```python
from build123d import *

# Parameters (mm, degrees)
SKETCH1_R               = 12.9794
BOSS_EXTRUDE1_DEPTH     = 25.4
CUT_EXTRUDE1_DEPTH      = 76.208452105
CUT_EXTRUDE1_DEPTH_BACK = 76.208452105
SKETCH3_R               = 3.81
SKETCH6_R               = 8.255
CUT_EXTRUDE2_DEPTH      = 2.032
SKETCH7_R               = 3.81
SKETCH7_R_2             = 1.905
CUT_EXTRUDE3_DEPTH      = 26.67
SKETCH7_3_R             = 1.905
CUT_EXTRUDE4_DEPTH      = 46.693656372


with BuildPart() as part:
    # Sketch1 → Boss-Extrude1 (new body)
    with BuildSketch(Plane(origin=(0, 0, 0), x_dir=(1, 0, 0), z_dir=(0, 1, 0))):
        with Locations(Location((0, 0, 0), (0, 0, 270))):
            Circle(SKETCH1_R)
    extrude(amount=BOSS_EXTRUDE1_DEPTH)

    # Sketch2 → Revolve1 (revolve)
    with BuildSketch(Plane(origin=(0, 0, 0), x_dir=(0, 0, -1), z_dir=(1, 0, 0))):
        with BuildLine():
            Line((-16.764, 25.4), (-16.764, 54.61))
            ThreePointArc((-16.764, 54.61), (-11.85393808, 66.46393808), (0, 71.374))
            Line((0, 71.374), (0, 25.4))
            Line((0, 25.4), (-16.764, 25.4))
        make_face()
    revolve(axis=Axis((0, 25.4, 0), (0, 1, 0)))

    # Sketch3 → Cut-Extrude1 (cut, two sides: drawn at the far end of the back side and taken through both)
    with BuildSketch(Plane(origin=(0, 0, 0), x_dir=(0, 0, -1), z_dir=(1, 0, 0)).offset(-CUT_EXTRUDE1_DEPTH_BACK)):
        with Locations((0, 54.61)):
            Circle(SKETCH3_R)
    extrude(amount=CUT_EXTRUDE1_DEPTH + CUT_EXTRUDE1_DEPTH_BACK, mode=Mode.SUBTRACT)

    # Sketch4 → Cut-Revolve1 (revolve, cut)
    with BuildSketch(Plane.XY, mode=Mode.PRIVATE) as cut_revolve1_sk:
        with BuildLine():
            Line((-7.62, 38.1), (-7.62, 54.61))
            Line((-7.62, 54.61), (7.62, 54.61))
            Line((7.62, 54.61), (7.62, 38.1))
            ThreePointArc((7.62, 38.1), (0, 36.42636725), (-7.62, 38.1))
        make_face()
    revolve(cut_revolve1_sk.sketch.rotate(Axis((-7.62, 54.61, 0), (1, 0, 0)), 90), axis=Axis((-7.62, 54.61, 0), (1, 0, 0)), mode=Mode.SUBTRACT)

    # Sketch6 → Cut-Extrude2 (cut)
    with BuildSketch(Plane(origin=(16.764, 0, 0), x_dir=(0, 0, -1), z_dir=(1, 0, 0))):
        with Locations((0, 54.61)):
            Circle(SKETCH6_R)
    cut_extrude2 = extrude(amount=-CUT_EXTRUDE2_DEPTH, mode=Mode.SUBTRACT)

    # Mirror1: Cut-Extrude2 across plane
    add(cut_extrude2.mirror(Plane(origin=(0, 0, 0), x_dir=(0, 0, 1), z_dir=(1, 0, 0))), mode=Mode.SUBTRACT)

    # Sketch7 → Cut-Extrude3 (cut)
    # profile 1 of 2: a face of its own
    with BuildSketch(Plane(origin=(0, 30.48, 0), x_dir=(1, 0, 0), z_dir=(0, 1, 0))):
        with Locations(Location((0, 0, 0), (0, 0, 270))):
            Circle(SKETCH7_R)
        Circle(SKETCH7_R_2, mode=Mode.SUBTRACT)
    # profile 2 of 2: a face of its own
    with BuildSketch(Plane(origin=(0, 30.48, 0), x_dir=(1, 0, 0), z_dir=(0, 1, 0))):
        Circle(SKETCH7_R_2)
    extrude(amount=CUT_EXTRUDE3_DEPTH, mode=Mode.SUBTRACT)

    # Sketch7_3 → Cut-Extrude4 (cut, through all)
    with BuildSketch(Plane(origin=(0, 30.48, 0), x_dir=(1, 0, 0), z_dir=(0, 1, 0))):
        with Locations(Location((0, 0, 0), (0, 0, 270))):
            Circle(SKETCH7_3_R)
    extrude(amount=-CUT_EXTRUDE4_DEPTH, mode=Mode.SUBTRACT)


solid = part.part
```
For this review, take the finished solid that the model builds, in its own axes (mm). A direction names the side the tool comes from. Round coordinates to 2 decimals unless told otherwise and drop trailing zeros. Loops run counter-clockwise (first coordinate to the right, second up) from the corner with the lowest first, then second, coordinate; pieces in that order, holes last.
(1) Tool access review of faces 4 (the flat face through (7.62, 50.5, -0.2)), 5 (the cylindrical face through (15.537, 46.356, 0.153)), 6 (the cylindrical face through (-15.537, 46.356, 0.153)), 7 (the flat face through (-10, 25.4, -9)): name each direction out of +Z, -Z, +X, -X, +Y, -Y from which nothing blocks a thin tool from reaching the whole face with its end or side.
Returned:
face 4: +Y
face 5: +X, +Y
face 6: -X, +Y
face 7: -Y
(2) We need section C-C (y = 57.5). Give the boundary of the cut face in (x, z).
Returned:
outline: (-14.73, -7.46) arc R16.51 ccw to (-7.62, -14.65) - (-7.62, -2.48) - (-14.73, -2.48) - close; (-14.73, 2.48) - (-7.62, 2.48) - (-7.62, 14.65) arc R16.51 ccw to (-14.73, 7.46) - close; (7.62, -14.65) arc R16.51 ccw to (14.73, -7.46) - (14.73, -2.48) - (7.62, -2.48) - close; (7.62, 2.48) - (14.73, 2.48) - (14.73, 7.46) arc R16.51 ccw to (7.62, 14.65) - close
(3) We need section A-A (z = 0). State how many separate pieces and enclosed holes the cut face has, plus the area to 3 significant figures.
Returned:
separate pieces: 4
enclosed holes: 0
area: 1,240 mm2
(4) Mouldability with a two-part tool opening along Z and no side actions: class faces 1 (the flat face through (-3, 0, 0)), 2 (the cylindrical face through (-11.226, 58.388, 0.496)), 3 (the cylindrical face through (-7.9, 12.5, -10.3)) as released by +Z, released by -Z, zero draft, split by the parting line, or undercut.
Returned:
face 1: zero draft
face 2: undercut
face 3: split by the parting line
(5) We need section D-D (y = 5). Give the boundary of the cut face in (x, z) (3 decimals).
Returned:
outline: circle Ø25.959 at (0, 0); hole circle Ø3.81 at (0, 0)
(6) Wall thickness on line 1 along X through (y, z) = (34.5, 0); line 2 along X through (y, z) = (48, 4): over which ranges is each line inside the solid? List them lowest first.
Returned:
line 1: x = -16.76 to -3.81, 3.81 to 16.76
line 2: x = -14.73 to -7.62, 7.62 to 14.73
(7) We need section B-B (x = 0). Give the boundary of the cut face in (y, z) (3 decimals).
Returned:
outline: (0, -12.979) - (25.4, -12.979) - (25.4, -16.764) - (47.566, -16.764) arc R18.184 cw to (36.83, -3.81) - (30.48, -3.81) - (30.48, -1.905) - (0, -1.905) - close; (0, 1.905) - (30.48, 1.905) - (30.48, 3.81) - (36.83, 3.81) arc R18.184 cw to (47.566, 16.764) - (25.4, 16.764) - (25.4, 12.979) - (0, 12.979) - close
(8) Clearance check with flat-ended pins moving along their axes: P1, Ø15, axis at y = 46, z = 5.5, coming from the -X side; P2, Ø1, axis at x = 4, y = 16, coming from the -Z side; P3, Ø3, axis at y = 27, z = -3, coming from the -X side; P4, Ø1.5, axis at x = 8.5, y = 62.5, coming from the +Z side. State where each tip first meets the part, or that it passes through.
Returned:
P1: stops at x = -16.76
P2: stops at z = -12.5
P3: stops at x = -16.7
P4: stops at z = 12.78
